Input: part model. Units: mm. Frame: model coordinates. Face numbers are marked on the shaded views. A direction names the side the tool comes from. Round coordinates to 2 decimals unless told otherwise and drop trailing zeros. Use CSV: the item, a comma, the result in double quotes. Start each with the question number.
1. Pull-direction query (Y, two-part tool) for the marked faces 1, 2 and 3; classes: +Y half, -Y half, draft (parallel to the pull), parting line (faces both ways), or undercut.
2. Access query for the marked faces 4, 5, 6 and 7. Directions: +Z, -Z, +X, -X, +Y, -Y. A direction counts if a zero-diameter tool reaches every point of the face in a straight line with its end or side. Return the directions, or none.
3. Material intervals for probe 1 along Y at (x, z) = (-17.25, 4.25); probe 2 along Y at (x, z) = (17.25, 4.25); probe 3 along Y at (x, z) = (-14.5, 4.75), sorted ascending. Write a range as from..to.
4. Pin query (flat end, axial travel): P1, Ø2.5, axis at x = -17.25, y = 30.75, coming from the -Z side; P2, Ø4, axis at x = 16.5, z = 3, coming from the +Y side; P3, Ø4, axis at y = 16.5, z = 3.5, coming from the -X side; P4, Ø4, axis at x = 10.5, y = -26.5, coming from the -Z side. Return the tip coordinate at first contact, or that it passes through.
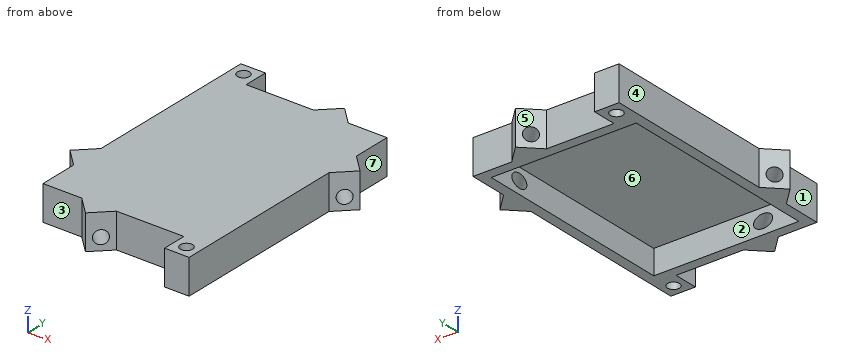
Autodesk Inventor part; units mm, degrees
ref_plane "YZ Plane" through (0, 0, 0) normal (1, 0, 0) x (0, 1, 0)
ref_plane "XZ Plane" through (0, 0, 0) normal (0, 1, 0) x (-1, 0, 0)
ref_plane "XY Plane" through (0, 0, 0) normal (0, 0, 1) x (1, 0, 0)
sketch "Skizze1" plane through (0, 0, 0) normal (0, 0, 1) x (1, 0, 0)
  line L0 (-17.75, -25.25) -> (17.75, -25.25)
  line L1 (17.75, -25.25) -> (17.75, 25.25)
  line L2 (17.75, 25.25) -> (-17.75, 25.25)
  line L3 (-17.75, 25.25) -> (-17.75, -25.25)
  line L4 (20.25, 27.75) -> (20.25, -27.75)
  line L5 (20.25, -27.75) -> (-20.25, -27.75)
  line L6 (-20.25, -27.75) -> (-20.25, 27.75)
  line L7 (-20.25, 27.75) -> (20.25, 27.75)
  point P0 (0, 0)
  point P1 (0, 25.25)
  point P2 (17.75, 0)
  dimension "d0" = 50.5
  dimension "d1" = 35.5
  dimension "d2" = 2.5
extrude "Extrusion1" [suppressed]
extrude "Extrusion2" add sketch "Skizze1" along normal blind 6
sketch "Skizze2" plane through (0, 0, -2.5) normal (0, 0, -1) x (-1, 0, 0)
  circle A0 centre (0, 0) radius 1.5
  dimension "d7" = 3
extrude "Extrusion3" [suppressed]
sketch "Skizze3" plane through (0, 0, 6) normal (0, 0, 1) x (1, 0, 0)
  line L0 (2.2647, 27.75) -> (10.75, 27.75)
  line L1 (10.75, 27.75) -> (6.5074, 31.9926)
  line L2 (6.5074, 31.9926) -> (2.2647, 27.75)
  line L3 (20.25, 18.25) -> (20.25, 9.7647)
  line L4 (20.25, 9.7647) -> (24.4926, 14.0074)
  line L5 (24.4926, 14.0074) -> (20.25, 18.25)
  line L6 (20.25, 27.75) -> (-20.25, 27.75)
  line L7 (20.25, -27.75) -> (20.25, 27.75)
  line L8 (4.386, 29.8713) -> (22.3713, 11.886) construction
  line L9 (-20.25, -9.7647) -> (-20.25, -18.25)
  line L10 (-20.25, -18.25) -> (-24.4926, -14.0074)
  line L11 (-24.4926, -14.0074) -> (-20.25, -9.7647)
  line L12 (-10.75, -27.75) -> (-2.2647, -27.75)
  line L13 (-2.2647, -27.75) -> (-6.5074, -31.9926)
  line L14 (-6.5074, -31.9926) -> (-10.75, -27.75)
  line L15 (-20.25, 27.75) -> (-20.25, -27.75)
  line L16 (-20.25, -27.75) -> (20.25, -27.75)
  line L17 (-22.3713, -11.886) -> (-4.386, -29.8713) construction
  line L18 (17.75, 25.25) -> (17.75, -25.25)
  line L19 (-17.75, -25.25) -> (-17.75, 25.25)
  line L20 (-17.75, 25.25) -> (17.75, 25.25)
  line L21 (17.75, -25.25) -> (-17.75, -25.25)
  point P0 (0, 0)
  dimension "d11" = 6
  dimension "d26" = 7
  dimension "d27" = 7
extrude "Extrusion4" add sketch "Skizze3" against normal blind 6 contours L2 L1 L0 | L9 L10 L11 | L5 L4 L3 | L12 L13 L14
sketch "Skizze4" plane through (6.5074, 31.9926, 0) normal (-0.7071, 0.7071, 0) x (-0.7071, -0.7071, 0)
  circle A0 centre (3, 3) radius 1.65
  line L0 (6, 0) -> (6, 6) construction
  line L1 (0, 6) -> (0, 0) construction
  line L2 (6, 0) -> (0, 0) construction
  line L3 (0, 0) -> (0, 6) construction
  line L4 (0, 6) -> (6, 6) construction
  line L5 (6, 6) -> (6, 0) construction
  point P0 (27.2236, 0)
  point P1 (0, 3)
  point P2 (3, 0)
  dimension "d28" = 3.3
extrude "Extrusion5" cut sketch "Skizze4" against normal up to surface (25.435 mm away)
sketch "Skizze7" plane through (-20.25, -9.7647, 0) normal (-0.7071, 0.7071, 0) x (-0.7071, -0.7071, 0)
  line L0 (0, 0) -> (0, 6) construction
  line L1 (6, 6) -> (6, 0) construction
  line L2 (0, 0) -> (6, 0) construction
  line L3 (6, 0) -> (6, 6) construction
  line L4 (6, 6) -> (0, 6) construction
  line L5 (0, 6) -> (0, 0) construction
  circle A0 centre (3, 3) radius 1.65
  point P0 (-21.2236, 0)
  point P1 (0, 3)
  point P2 (3, 6)
  dimension "d29" = 3.3
extrude "Extrusion8" cut sketch "Skizze7" against normal up to surface (25.435 mm away)
sketch "Skizze8" plane through (0, 0, 6) normal (0, 0, 1) x (1, 0, 0)
  line L0 (-20.25, 27.75) -> (2.2647, 27.75)
  line L1 (-20.25, 27.75) -> (-20.25, -9.7647)
  line L2 (-20.25, -9.7647) -> (-24.4926, -14.0074)
  line L3 (-20.25, -9.7647) -> (-24.4926, -14.0074)
  line L4 (-24.4926, -14.0074) -> (-20.25, -18.25)
  line L5 (-10.75, -27.75) -> (-20.25, -27.75)
  line L6 (-20.25, -18.25) -> (-20.25, -27.75)
  line L7 (-20.25, -27.75) -> (-10.75, -27.75)
  line L8 (-10.75, -27.75) -> (-6.5074, -31.9926)
  line L9 (-10.75, -27.75) -> (-6.5074, -31.9926)
  line L10 (-2.2647, -27.75) -> (-6.5074, -31.9926)
  line L11 (-6.5074, -31.9926) -> (-2.2647, -27.75)
  line L12 (-2.2647, -27.75) -> (20.25, -27.75)
  line L13 (-2.2647, -27.75) -> (20.25, -27.75)
  line L14 (20.25, 9.7647) -> (20.25, -27.75)
  line L15 (20.25, -27.75) -> (20.25, 9.7647)
  line L16 (24.4926, 14.0074) -> (20.25, 9.7647)
  line L17 (20.25, 9.7647) -> (24.4926, 14.0074)
  line L18 (20.25, 27.75) -> (20.25, 18.25)
  line L19 (24.4926, 14.0074) -> (20.25, 18.25)
  line L20 (20.25, 18.25) -> (20.25, 27.75)
  line L21 (10.75, 27.75) -> (20.25, 27.75)
  line L22 (20.25, 27.75) -> (10.75, 27.75)
  line L23 (2.2647, 27.75) -> (6.5074, 31.9926)
  line L24 (10.75, 27.75) -> (6.5074, 31.9926)
  line L25 (6.5074, 31.9926) -> (2.2647, 27.75)
  line L26 (2.2647, 27.75) -> (-20.25, 27.75)
  point P0 (0, 0)
extrude "Extrusion9" add sketch "Skizze8" along normal blind 2.5
sketch "Skizze11" plane through (0, 0, 8.5) normal (0, 0, 1) x (1, 0, 0)
  line L0 (-10.75, -27.75) -> (-20.25, -27.75) construction
  line L1 (20.25, 27.75) -> (20.25, 18.25) construction
  line L2 (-20.25, 27.75) -> (2.2647, 27.75)
  line L3 (-20.25, 27.75) -> (-14.25, 27.75)
  line L4 (-14.25, 27.75) -> (-14.25, 33.75)
  line L5 (-14.25, 33.75) -> (-20.25, 33.75)
  line L6 (-20.25, 33.75) -> (-20.25, 27.75)
  circle A0 centre (-17.25, 30.75) radius 1.5
  line L7 (20.25, -27.75) -> (-2.2647, -27.75)
  line L8 (20.25, -27.75) -> (14.25, -27.75)
  line L9 (14.25, -27.75) -> (14.25, -33.75)
  line L10 (14.25, -33.75) -> (20.25, -33.75)
  line L11 (20.25, -33.75) -> (20.25, -27.75)
  circle A1 centre (17.25, -30.75) radius 1.5
  point P0 (0, 0)
  point P1 (-20.25, 30.75)
  point P2 (-17.25, 33.75)
  point P3 (17.25, -27.75)
  point P4 (20.25, -30.75)
  dimension "d42" = 6
  dimension "d43" = 3
extrude "Extrusion12" add sketch "Skizze11" against normal up to surface (8.5 mm away)
equation "\"d27\" = d26"
properties part number "cage"
Established:
1,face 1,"draft"
1,face 2,"undercut"
1,face 3,"-Y half"
2,face 4,"+Z, -Z, -X, +Y"
2,face 5,"+Z, -Z, +Y"
2,face 6,"-Z"
2,face 7,"+Z, -Z, +X, +Y"
3,probe 1,"y = -27.75..-25.25, 25.25..29.25, 32.25..33.75"
3,probe 2,"y = -33.75..-32.25, -29.25..-25.25, 25.25..27.75"
3,probe 3,"y = -27.75..-25.25, 25.25..33.75"
4,P1,"passes through"
4,P2,"stops at y = 27.75"
4,P3,"stops at x = -20.25"
4,P4,"stops at z = 0"
